from build123d import *

# Parameters (mm, degrees)
CROQUIS1_W               = 22
CROQUIS1_H               = 55.2
SALIENTE_EXTRUIR1_DEPTH  = 4
CROQUIS2_W               = 12.1
CROQUIS2_H               = 4
CORTAR_EXTRUIR1_DEPTH    = 9.6
CROQUIS3_W               = 12.1
CROQUIS3_H               = 4
CORTAR_EXTRUIR2_DEPTH    = 9.6
CORTAR_EXTRUIR3_DEPTH    = 16
CORTAR_EXTRUIR4_START    = -16
CORTAR_EXTRUIR4_DEPTH    = 16
CROQUIS9_W               = 11.778481694
CROQUIS9_H               = 4
CORTAR_EXTRUIR5_DEPTH    = 2
CROQUIS11_W              = 4.95
CROQUIS11_H              = 4
SALIENTE_EXTRUIR3_DEPTH  = 2
CROQUIS12_W              = 4
CROQUIS12_H              = 1.8
SALIENTE_EXTRUIR4_DEPTH  = 12.1
CROQUIS13_W              = 4.95
CROQUIS13_H              = 4
SALIENTE_EXTRUIR5_DEPTH  = 2
CROQUIS14_W              = 4
CROQUIS14_H              = 1.8
SALIENTE_EXTRUIR6_DEPTH  = 12.1
CROQUIS17_W              = 4
CROQUIS17_H              = 59.2
SALIENTE_EXTRUIR8_DEPTH  = 23
CROQUIS18_W              = 4
CROQUIS18_H              = 59.2
SALIENTE_EXTRUIR9_DEPTH  = 23
CROQUIS19_R              = 1.75
CORTAR_EXTRUIR6_DEPTH    = 11.5
CROQUIS20_R              = 8.8
CROQUIS20_R_2            = 8.901027098
CORTAR_EXTRUIR7_DEPTH    = 4
CORTAR_EXTRUIR8_DEPTH    = 10
CROQUIS22_R              = 10
CROQUIS22_R_2            = 8
SALIENTE_EXTRUIR10_DEPTH = 6


with BuildPart() as part:
    # Croquis1 → Saliente-Extruir1 (new body)
    with BuildSketch(Plane.XY):
        with Locations((11, 27.6)):
            Rectangle(CROQUIS1_W, CROQUIS1_H)
    extrude(amount=SALIENTE_EXTRUIR1_DEPTH)

    # Croquis2 → Cortar-Extruir1 (cut)
    with BuildSketch(Plane(origin=(0, 55.2, 0), x_dir=(1, 0, 0), z_dir=(0, 1, 0))):
        with Locations((11, -2)):
            Rectangle(CROQUIS2_W, CROQUIS2_H)
    extrude(amount=-CORTAR_EXTRUIR1_DEPTH, mode=Mode.SUBTRACT)

    # Croquis3 → Cortar-Extruir2 (cut)
    with BuildSketch(Plane.XZ):
        with Locations((11, 2)):
            Rectangle(CROQUIS3_W, CROQUIS3_H)
    extrude(amount=-CORTAR_EXTRUIR2_DEPTH, mode=Mode.SUBTRACT)

    # Croquis5 → Cortar-Extruir3 (cut)
    with BuildSketch(Plane.XZ.offset(-9.6)):
        with BuildLine():
            Line((7.4, 4), (14.6, 4))
            ThreePointArc((14.6, 4), (16.401151853, 1.506649462), (17.05, -1.5))
            Line((17.05, -1.5), (4.95, -1.5))
            ThreePointArc((4.95, -1.5), (5.598848147, 1.506649462), (7.4, 4))
        make_face()
    extrude(amount=-CORTAR_EXTRUIR3_DEPTH, mode=Mode.SUBTRACT)

    # Croquis7 → Cortar-Extruir4 (cut)
    with BuildSketch(Plane(origin=(0, 45.6, 0), x_dir=(1, 0, 0), z_dir=(0, 1, 0)).offset(CORTAR_EXTRUIR4_START)):
        with BuildLine():
            Line((4.95, 1.5), (17.05, 1.5))
            ThreePointArc((17.05, 1.5), (16.401151853, -1.506649462), (14.6, -4))
            Line((14.6, -4), (7.4, -4))
            ThreePointArc((7.4, -4), (5.598848147, -1.506649462), (4.95, 1.5))
        make_face()
    extrude(amount=CORTAR_EXTRUIR4_DEPTH, mode=Mode.SUBTRACT)

    # Croquis9 → Cortar-Extruir5 (cut)
    with BuildSketch(Plane(origin=(0, 0, 0), x_dir=(-1, 0, 0), z_dir=(0, 0, -1))):
        with Locations((-11, 27.6)):
            Rectangle(CROQUIS9_W, CROQUIS9_H)
    extrude(amount=-CORTAR_EXTRUIR5_DEPTH, mode=Mode.SUBTRACT)

    # Croquis11 → Saliente-Extruir3 (add)
    with BuildSketch(Plane(origin=(0, 55.2, 0), x_dir=(1, 0, 0), z_dir=(0, 1, 0))):
        with Locations((2.475, -2)):
            Rectangle(CROQUIS11_W, CROQUIS11_H)
        with Locations((19.525, -2)):
            Rectangle(CROQUIS11_W, CROQUIS11_H)
    extrude(amount=SALIENTE_EXTRUIR3_DEPTH)

    # Croquis12 → Saliente-Extruir4 (add)
    with BuildSketch(Plane(origin=(4.95, 0, 0), x_dir=(0, 0, -1), z_dir=(1, 0, 0))):
        with Locations((-2, 56.3)):
            Rectangle(CROQUIS12_W, CROQUIS12_H)
    extrude(amount=SALIENTE_EXTRUIR4_DEPTH)

    # Croquis13 → Saliente-Extruir5 (add)
    with BuildSketch(Plane.XZ):
        with Locations((19.525, 2)):
            Rectangle(CROQUIS13_W, CROQUIS13_H)
        with Locations((2.475, 2)):
            Rectangle(CROQUIS13_W, CROQUIS13_H)
    extrude(amount=SALIENTE_EXTRUIR5_DEPTH)

    # Croquis14 → Saliente-Extruir6 (add)
    with BuildSketch(Plane(origin=(4.95, 0, 0), x_dir=(0, 0, -1), z_dir=(1, 0, 0))):
        with Locations((-2, -1.1)):
            Rectangle(CROQUIS14_W, CROQUIS14_H)
    extrude(amount=SALIENTE_EXTRUIR6_DEPTH)

    # Croquis17 → Saliente-Extruir8 (add)
    with BuildSketch(Plane.ZY):
        with Locations((2, 27.6)):
            Rectangle(CROQUIS17_W, CROQUIS17_H)
    extrude(amount=SALIENTE_EXTRUIR8_DEPTH)

    # Croquis18 → Saliente-Extruir9 (add)
    with BuildSketch(Plane(origin=(22, 0, 0), x_dir=(0, 0, -1), z_dir=(1, 0, 0))):
        with Locations((-2, 27.6)):
            Rectangle(CROQUIS18_W, CROQUIS18_H)
    extrude(amount=SALIENTE_EXTRUIR9_DEPTH)

    # Croquis19 → Cortar-Extruir6 (cut)
    with BuildSketch(Plane(origin=(0, 0, 0), x_dir=(-1, 0, 0), z_dir=(0, 0, -1))):
        with Locations((-23.2, 54.9)):
            Circle(CROQUIS19_R)
        with Locations((1.2, 54)):
            Circle(CROQUIS19_R)
        with Locations((1.2, 0.5)):
            Circle(CROQUIS19_R)
        with Locations((-23.2, 0.5)):
            Circle(CROQUIS19_R)
    extrude(amount=-CORTAR_EXTRUIR6_DEPTH, mode=Mode.SUBTRACT)

    # Croquis20 → Cortar-Extruir7 (cut)
    with BuildSketch(Plane(origin=(0, 0, 0), x_dir=(-1, 0, 0), z_dir=(0, 0, -1))):
        with Locations((13, 27.6)):
            Circle(CROQUIS20_R)
        with Locations((-35, 27.6)):
            Circle(CROQUIS20_R_2)
    extrude(amount=-CORTAR_EXTRUIR7_DEPTH, mode=Mode.SUBTRACT)

    # Croquis21 → Cortar-Extruir8 (cut)
    with BuildSketch(Plane(origin=(0, 0, 0), x_dir=(-1, 0, 0), z_dir=(0, 0, -1))):
        Polygon((-45, 57.2), (-45, 34.2), (-27, 57.2), align=None)
        Polygon((-45, -2), (-45, 21), (-27, -2), align=None)
        Polygon((23, 57.2), (23, 34.2), (5, 57.2), align=None)
        Polygon((23, -2), (23, 21), (5, -2), align=None)
    extrude(amount=-CORTAR_EXTRUIR8_DEPTH, mode=Mode.SUBTRACT)

    # Croquis22 → Saliente-Extruir10 (add)
    # profile 1 of 2: a face of its own
    with BuildSketch(Plane.XY.offset(4)):
        with Locations((35, 27.6)):
            Circle(CROQUIS22_R)
        with Locations((35, 27.6)):
            Circle(CROQUIS22_R_2, mode=Mode.SUBTRACT)
    # profile 2 of 2: a face of its own
    with BuildSketch(Plane.XY.offset(4)):
        with Locations(Location((-13, 27.6, 0), (0, 0, 180))):
            Circle(CROQUIS22_R)
        with Locations((-13, 27.6)):
            Circle(CROQUIS22_R_2, mode=Mode.SUBTRACT)
    extrude(amount=SALIENTE_EXTRUIR10_DEPTH)

    # Croquis23 → Cortar-Revolución1 (revolve, cut)
    with BuildSketch(Plane.XY.offset(6)):
        with BuildLine():
            Line((43.8, 27.6), (26.2, 27.6))
            ThreePointArc((26.2, 27.6), (35, 36.4), (43.8, 27.6))
        make_face()
    revolve(axis=Axis((43.8, 27.6, 6), (-1, 0, 0)), mode=Mode.SUBTRACT)

    # Croquis24 → Cortar-Revolución2 (revolve, cut)
    with BuildSketch(Plane.XY.offset(6)):
        with BuildLine():
            Line((-13, 36.4), (-13, 18.8))
            ThreePointArc((-13, 18.8), (-21.8, 27.6), (-13, 36.4))
        make_face()
    revolve(axis=Axis((-13, 36.4, 6), (0, -1, 0)), mode=Mode.SUBTRACT)


solid = part.part
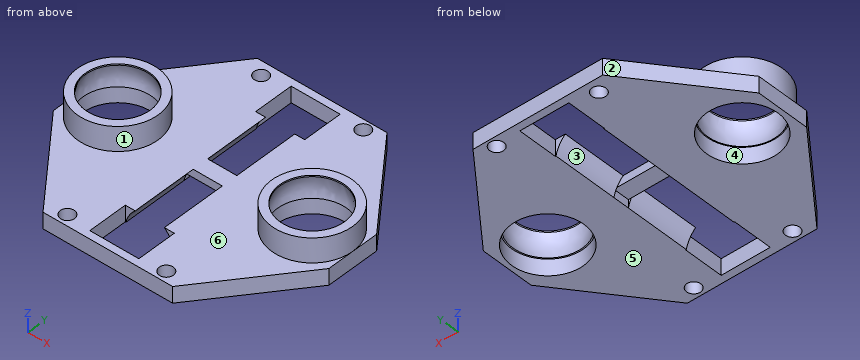
Read the model definition and answer for the solid it produces. Units are mm, in the model's axes. Face numbers are marked on the shaded views. A direction names the side the tool comes from. Coordinates: 2 decimals unless noted, no trailing zeros. Loops run counter-clockwise (first coordinate to the right, second up) from the corner with the lowest first, then second, coordinate; pieces in that order, holes last. Notation, with made-up numbers: (66.25, 72) - (82.25, 72) arc R29 cw to (82.25, 98) - close; hole circle Ø2 at (-25.75, 85.5). An arc over 180 degrees is marked (long way). Answer in a Markdown table with one row per item.
Q1. Find section B-B on x = -8.5. Write down the section's boundary in (y, z), plus the area to 3 significant figures.
Here are the results:
| item | result |
|---|---|
| outline | (2.47, 0) - (20.04, 0) - (20.04, 4) - (20.31, 4) arc R7.56 cw to (20.99, 9.67) - (20.99, 10) - (18.67, 10) - (18.67, 4) - (2.47, 4) - close; (34.21, 9.67) arc R7.56 cw to (34.89, 4) - (35.16, 4) - (35.16, 0) - (52.73, 0) - (52.73, 4) - (36.53, 4) - (36.53, 10) - (34.21, 10) - close |
| area | 160 mm^2 |
Q2. Given P1, Ø3, axis at x = 37, y = 44.5, coming from the -Z side; P2, Ø2, axis at x = -12, z = 2, coming from the +Y side; P3, Ø1.5, axis at x = 15, y = 47.5, coming from the +Z side; P4, Ø1.2, axis at y = 49, z = 2, coming from the -X side, each flat-ended and moving along its own axis, determine where each tip first touches the part or whether it passes through.
Here are the results:
| item | result |
|---|---|
| P1 | stops at z = 0 |
| P2 | stops at y = 49.53 |
| P3 | passes through |
| P4 | stops at x = -11.89 |
Q3. Find section C-C on z = 7. Write down the section's boundary in (x, y), plus the area to 3 significant figures.
Here are the results:
| item | result |
|---|---|
| outline | circle Ø20 at (-13, 27.6); circle Ø20 at (35, 27.6); hole circle Ø17.49 at (-13, 27.6); hole circle Ø17.49 at (35, 27.6) |
| area | 148 mm^2 |
Q4. Straight lines are drawn through the part: line 1 along Y through (x, z) = (23.2, 0.9); line 2 along Y through (x, z) = (-1.2, 2); line 3 along X through (y, z) = (34, 4.75). For each, find the intervals that lie inside material, in ascending order. Write a range as [from, to].
Here are the results:
| item | result |
|---|---|
| line 1 | y = [-2, -1.25], [2.25, 53.15], [56.65, 57.2] |
| line 2 | y = [-2, -1.25], [2.25, 52.25], [55.75, 57.2] |
| line 3 | x = [-20.68, -18.91], [-7.09, -5.32], [27.32, 29.09], [40.91, 42.68] |
Q5. Find section D-D on y = 54. Write down the section's boundary in (x, z).
Here are the results:
| item | result |
|---|---|
| outline | (-7.5, 0) - (-2.95, 0) - (-2.95, 4) - (-7.5, 4) - close; (0.55, 0) - (4.95, 0) - (4.95, 4) - (0.55, 4) - close; (17.05, 0) - (21.7, 0) - (21.7, 4) - (17.05, 4) - close; (24.7, 0) - (29.5, 0) - (29.5, 4) - (24.7, 4) - close |
Q6. The mould has two halves that part along Y. Classify the marked faces 1, 2 and 3: pulls with the +Y half, pulls with the -Y half, needs draft (parallel to the pull), parting line crosses it, or undercut.
Here are the results:
| item | result |
|---|---|
| face 1 | parting line crosses it |
| face 2 | pulls with the +Y half |
| face 3 | undercut |
Q7. For the marked faces 4, 5 and 6, determine the directions among +Z, -Z, +X, -X, +Y, -Y from which every point of the face is accessible in a straight line to the end or side of a thin tool.
Here are the results:
| item | result |
|---|---|
| face 4 | -Z |
| face 5 | -Z, +X, -X, +Y, -Y |
| face 6 | +Z |
Q8. Find section A-A on y = 14. Write down the section's boundary in (x, z).
Here are the results:
| item | result |
|---|---|
| outline | (-17.52, 0) - (5.11, 0) arc R7.5 cw to (7.4, 4) - (-17.52, 4) - close; (14.6, 4) arc R7.5 cw to (16.89, 0) - (39.52, 0) - (39.52, 4) - close |
